```python
from build123d import *

# Parameters (mm, degrees)
SKETCH1_R           = 1.5
BOSS_EXTRUDE1_DEPTH = 20
FILLET1_R           = 0.3
FILLET2_R           = 0.2


with BuildPart() as part:
    # Sketch1 → Boss-Extrude1 (new body)
    with BuildSketch(Plane.XY):
        Polygon((3, 0), (1.5, 2.598076211), (-1.5, 2.598076211), (-3, 0), (-1.5, -2.598076211), (1.5, -2.598076211), align=None)
        Circle(SKETCH1_R, mode=Mode.SUBTRACT)
    extrude(amount=BOSS_EXTRUDE1_DEPTH)

    # Fillet1
    fillet1_edges = [part.edges().sort_by_distance(p)[0] for p in [
        (-1.5, 0, 0),
        (-1.5, 0, 20),
    ]]
    fillet(fillet1_edges, radius=FILLET1_R)

    # Fillet2
    fillet2_edges = [part.edges().sort_by_distance(p)[0] for p in [
        (0, 2.598076211, 20),
        (-2.25, 1.299038106, 20),
        (-2.25, -1.299038106, 20),
        (0, -2.598076211, 20),
        (2.25, -1.299038106, 20),
        (0, -2.598076211, 0),
        (-2.25, -1.299038106, 0),
        (-2.25, 1.299038106, 0),
        (2.25, 1.299038106, 20),
        (0, 2.598076211, 0),
        (2.25, 1.299038106, 0),
        (2.25, -1.299038106, 0),
    ]]
    fillet(fillet2_edges, radius=FILLET2_R)


solid = part.part
```
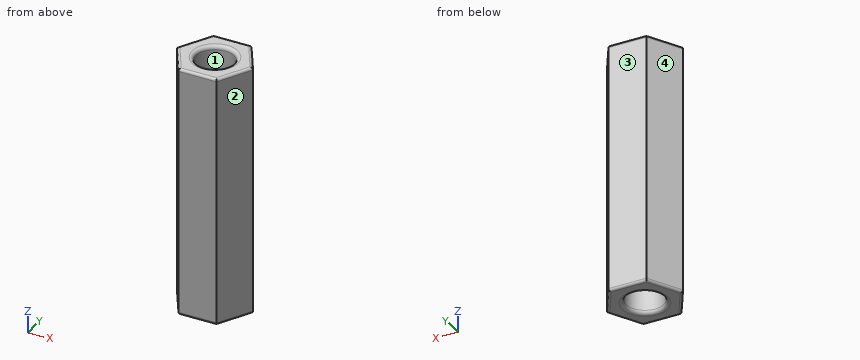
Can you work these out from the model? Positions are in its coordinate system, mm. Face numbers are marked on the shaded views. Coordinates: 2 decimals unless noted, no trailing zeros. Write each loop counter-clockwise with the first axis right and the second up, starting at its lowest first coordinate (ties: lowest second). Pieces come first, ordered by that corner, then holes. Notation, with made-up numbers: M 75,6.5 L 86,6.5 A27 ccw 86,36.5 Z; hole C 47.5,88 d7. An arc over 180 degrees is marked long. Write item = value, one per line. Start each with the question number.
Q1. If we section it at B-B, the plane x = 0: Write out the boundary of the cut face in (y, z).
Q2. If I drill on L1, parallel to Y at x = 0, z = 5.75; L2, parallel to X at y = 0.2, z = 18.5; L3, parallel to Z at x = 1.75, y = -0.25, over which ranges is the centre line in solid material (lowest first)? Write a range as [from, to].
Q3. I'm going to push flat-ended pins straight in: pin 1 (1.5 mm diameter, centred on y = 2, z = 4.5, fed in from +X); pin 2 (1.5 mm diameter, centred on y = -1, z = 7.5, fed in from +X); pin 3 (1 mm diameter, centred on y = -1, z = 6.5, fed in from -X). Where does each tip first touch, or does it pass through?
Q4. If we section it at A-A, the plane z = 9.75: Write out the boundary of the cut face in (x, y), then the cut area to 3 significant figures.
Q5. Thinking about a two-plate mould opening in X: for the marked faces 1, 2, 3 and 4, which applies, released by +X, released by -X, zero draft, split by the parting line, or undercut?
Check sheet entries:
q1.outline = M -2.6,0.2 A0.2 ccw -2.4,0 L -1.8,0 A0.3 ccw -1.5,0.3 L -1.5,19.7 A0.3 ccw -1.8,20 L -2.4,20 A0.2 ccw -2.6,19.8 Z; M 1.5,0.3 A0.3 ccw 1.8,0 L 2.4,0 A0.2 ccw 2.6,0.2 L 2.6,19.8 A0.2 ccw 2.4,20 L 1.8,20 A0.3 ccw 1.5,19.7 Z
q2.L1 = [-2.6, -1.5], [1.5, 2.6]
q2.L2 = [-2.88, -1.49], [1.49, 2.88]
q2.L3 = [0, 20]
q3.pin_1 = 2.28
q3.pin_2 = 2.86
q3.pin_3 = -2.71
q4.outline = M -3,0 L -1.5,-2.6 L 1.5,-2.6 L 3,0 L 1.5,2.6 L -1.5,2.6 Z; hole C 0,0 d3
q4.area = 16.3 mm²
q5.face_1 = undercut
q5.face_2 = released by +X
q5.face_3 = zero draft
q5.face_4 = released by -X
